Autodesk Inventor part; units mm, degrees
ref_plane "YZ Plane" through (0, 0, 0) normal (1, 0, 0) x (0, 1, 0)
ref_plane "XZ Plane" through (0, 0, 0) normal (0, 1, 0) x (-1, 0, 0)
ref_plane "XY Plane" through (0, 0, 0) normal (0, 0, 1) x (1, 0, 0)
sketch "Sketch4" plane through (0, 0, 0) normal (0, 0, 1) x (1, 0, 0)
  line L0 (-2.1, 0) -> (8, 0)
  line L1 (0, 0) -> (-2.1, 0)
  line L2 (0, 2.5) -> (0, 1.625)
  line L3 (0.4, 1.225) -> (0.4, 1.225)
  line L4 (0.4, 1.225) -> (0.8, 1.25)
  arc A0 (0, 1.625) -> (0.4, 1.225) centre (0.4, 1.625) ccw
  line L5 (-2.1, 0) -> (-2.1, 1.25)
  line L6 (0, 2.5) -> (-1.1375, 2.5)
  arc A1 (-1.1375, 2.5) -> (-2.1, 1.25) centre (1.4883, -0.5175) ccw
  line L7 (0.8, 1.25) -> (8, 1.25)
  line L8 (8, 1.25) -> (8, 0)
  point P0 (0, 1.225)
  dimension "d71" = 0.4
  dimension "d72" = 8
  dimension "d74" = 0.4
  dimension "d75" = 2.45
  dimension "d78" = 2.5
  dimension "d82" = 4
  dimension "d83" = 2.1
  dimension "d84" = 5
  dimension "d104" = 7.2
  dimension "d105" = 2.5
revolve "Revolution7" add sketch "Sketch4" angle 360 about axis through (-2.1, 0, 0) along (1, 0, 0)
sketch "Sketch5" plane through (-2.1, 0, 0) normal (-1, 0, 0) x (0, 0, 1)
  circle A0 centre (0, 0) radius 1.2 construction
  circle A1 centre (0, 0) radius 0.84 construction
  line L0 (0, 0) -> (-0.7275, 0.42)
  line L1 (0, 0) -> (-0.7275, -0.42)
  line L2 (-1.8008, 0) -> (1.7887, 0)
  line L3 (-1.2, 0) -> (-0.7275, -0.42)
  line L4 (-1.2, 0) -> (-0.7275, 0.42)
  dimension "d88" = 2.4
  dimension "d89" = 1.68
  dimension "d90" = 30
  dimension "d91" = 30
extrude "Extrusion1" cut sketch "Sketch5" against normal blind 1.04
pattern_circular "Circular Pattern1" count 6 over 360 about axis through (-10, 0, 0) along (1, 0, 0) of "Extrusion1"
fillet "Fillet1" radius 0.24 12 edges at (-1.58, -1.0392, -0.6) (-1.58, -0.42, -0.7275) (-1.58, -0.84, 0) (-1.58, -1.0392, 0.6) (-1.58, -0.42, 0.7275) (-1.58, 0, 1.2) (-1.58, 0.84, 0) (-1.58, 1.0392, 0.6) (-1.58, 0.42, 0.7275) (-1.58, 0.42, -0.7275) (-1.58, 0, -1.2) (-1.58, 1.0392, -0.6)
thread "Thread7"
properties part number "Flachkopfschraube mit Innenrund ISO 14583 - M2,5 x 8 - A3-70" material "Edelstahl"
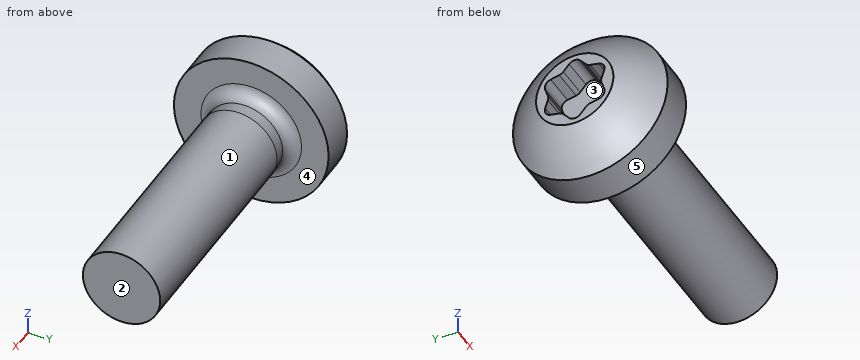
For this review, take the finished solid that the model builds, in its own axes (mm). Face numbers are marked on the shaded views. A direction names the side the tool comes from. Round coordinates to 2 decimals unless told otherwise and drop trailing zeros. Write each loop counter-clockwise with the first axis right and the second up, starting at its lowest first coordinate (ties: lowest second). Pieces come first, ordered by that corner, then holes. Notation, with made-up numbers: (61, 89.25) - (90, 89.25) arc R21 ccw to (90, 120.25) - close; hole circle Ø5 at (-26.75, -16). An arc over 180 degrees is marked (long way). Write item = value, one per line. Start each with the question number.
1. For pin 1 Ø2 at (x, z) = (3.5, -2) entering from +Y; pin 2 Ø1 at (x, y) = (1.5, 1) entering from +Z, all flat-tipped, find the tip position at first contact; note any pin that passes through.
2. Consider section A-A on x = 7. State the section outline as (y, z) points, plus the area to 3 significant figures.
3. Wall thickness on L1, parallel to X at y = -0.3, z = -0.4; L2, parallel to Y at x = 4.5, z = -0.6; L3, parallel to Y at x = -0.75, z = -2.1: over which ranges is each line inside the solid? List them lowest first.
4. Draft analysis for pull direction Z (two halves, no side actions). For the marked faces 3, 4 and 5, state which applies: released by +Z, released by -Z, zero draft, split by the parting line, or undercut.
5. Consider section B-B on x = 0.5. State the section outline as (y, z) points, plus the area to 3 significant figures.
6. For the marked faces 1 and 2, list the 3-axis set-ups (+Z, -Z, +X, -X, +Y, -Y) from which the entire face can be reached by the end or side of a thin tool; tool diameter is ignored.
Evaluation:
q1.pin_1 = 0.75
q1.pin_2 = 1.15
q2.outline = circle Ø2.5 at (0, 0)
q2.area = 4.91 mm2
q3.L1 = -1.06 to 8
q3.L2 = -1.1 to 1.1
q3.L3 = -1.36 to 1.36
q4.face_3 = undercut
q4.face_4 = zero draft
q4.face_5 = split by the parting line
q5.outline = circle Ø2.46 at (0, 0)
q5.area = 4.76 mm2
q6.face_1 = +X
q6.face_2 = +Z, -Z, +X, +Y, -Y
